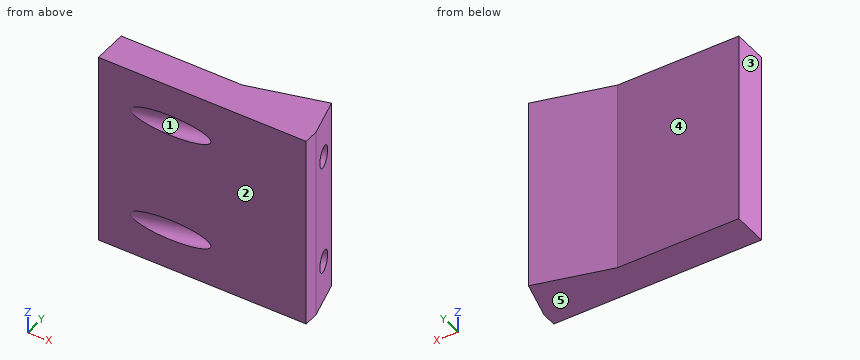
from build123d import *

# Parameters (mm, degrees)
BOSS_EXTRUDE1_DEPTH          = 44.45
F_3_8_0_375_DIAMETER_HOLE1_D = 9.525


with BuildPart() as part:
    # Sketch1 → Boss-Extrude1 (new, symmetric)
    with BuildSketch(Plane.XY):
        Polygon((95.25, 0), (95.25, 6.787222338), (90.319497191, 25.188109329), (55.5625, 15.875), (0, 15.875), (0, 0), align=None)
    extrude(amount=BOSS_EXTRUDE1_DEPTH, both=True)

    # 3/8 (0.375) Diameter Hole1 (through all)
    with Locations(Plane(origin=(90.56626544, 24.267157686, 0), x_dir=(0, 0, -1), z_dir=(0.9659258262890682, 0.2588190451025212, 0))):
        with Locations((-25.4, -8.571560701), (25.4, -8.571560701)):
            Hole(F_3_8_0_375_DIAMETER_HOLE1_D / 2)


solid = part.part
Design review of the part built by this model. Coordinates are the model's own, in mm. Face numbers are marked on the shaded views. A direction names the side the tool comes from. Coordinates: 2 decimals unless noted, no trailing zeros. Use one line per item in the form item = value.
Q1. Machinability: for the marked faces 4 and 5, which of the approach directions +Z, -Z, +X, -X, +Y, -Y give a long, thin tool a straight path to every point of the face, cutting with its end or side? Answer none if there is none.
Taken from the geometry:
face_4 = +Z, -Z, -X, +Y
face_5 = -Z, +X, -X, +Y, -Y
Q2. Consider section C-C (y = 9.25). Count the separate pieces of the cut face and the enclosed holes in it, plus the area to 3 significant figures.
Taken from the geometry:
separate_pieces = 1
enclosed_holes = 2
area = 7,860 mm^2
Q3. Insertion check: pin 1 Ø5 at (x, z) = (66.5, -35) entering from +Y; pin 2 Ø2 at (y, z) = (13, 16) entering from +X; pin 3 Ø6 at (y, z) = (18.5, 23) entering from +X. Each pin has a flat end and moves straight along its axis. Give the tip position at first contact, or say it passes through.
Taken from the geometry:
pin_1 = 19.48
pin_2 = 93.85
pin_3 = 92.62
Q4. For probe 1 along Z at (x, y) = (45, 4.75); probe 2 along Z at (x, y) = (83, 16.75); probe 3 along Y at (x, z) = (58.5, -24), list the stretches that pass through material, from the lowest coordinate up.
Taken from the geometry:
probe_1 = -44.45 to -29.92, -20.88 to 20.88, 29.92 to 44.45
probe_2 = -44.45 to -28.86, -21.94 to 21.94, 28.86 to 44.45
probe_3 = 0 to 2.09, 11.51 to 16.66
Q5. The part is to be moulded in two halves that separate along X. For the marked faces 1, 2 and 3, say which applies: +X half, -X half, draft (parallel to the pull), parting line (faces both ways), or undercut.
Taken from the geometry:
face_1 = undercut
face_2 = draft
face_3 = -X half
